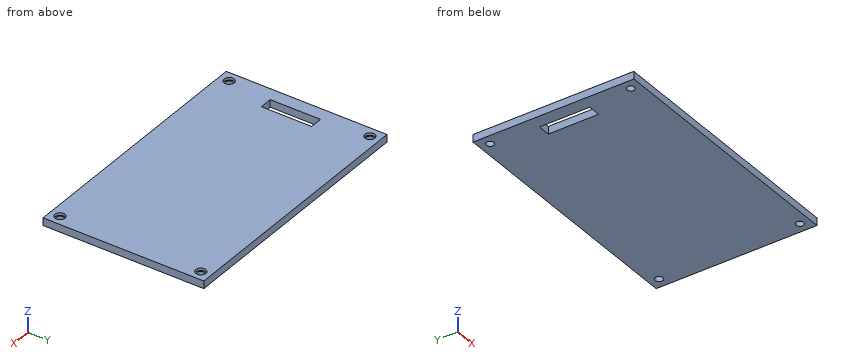
from build123d import *

# Parameters (mm, degrees)
SKETCH_1_W          = 104
SKETCH_1_H          = 64
EXTRUDE_1_DEPTH     = 3
SKETCH_2_R          = 1.5
CUT_EXTRUDE_1_DEPTH = 62.131006862
SKETCH_3_W          = 5
SKETCH_3_H          = 20
CUT_EXTRUDE_2_DEPTH = 62.131006862
SKETCH_4_R          = 2
CUT_EXTRUDE_3_DEPTH = 1


with BuildPart() as part:
    # 草图1 → 凸台-拉伸1 (new body)
    with BuildSketch(Plane.XY):
        Rectangle(SKETCH_1_W, SKETCH_1_H)
    extrude(amount=EXTRUDE_1_DEPTH)

    # 草图2 → 切除-拉伸1 (cut, through all)
    with BuildSketch(Plane.XY.offset(3)):
        with Locations((-48, 28)):
            Circle(SKETCH_2_R)
        with Locations(Location((48, 28, 0), (0, 0, 180))):
            Circle(SKETCH_2_R)
        with Locations((48, -28)):
            Circle(SKETCH_2_R)
        with Locations(Location((-48, -28, 0), (0, 0, 180))):
            Circle(SKETCH_2_R)
    extrude(amount=-CUT_EXTRUDE_1_DEPTH, mode=Mode.SUBTRACT)

    # 草图3 → 切除-拉伸2 (cut, through all)
    with BuildSketch(Plane(origin=(0, 0, 0), x_dir=(-1, 0, 0), z_dir=(0, 0, -1))):
        with Locations((44.26005687, -0.800014708)):
            Rectangle(SKETCH_3_W, SKETCH_3_H)
    extrude(amount=-CUT_EXTRUDE_2_DEPTH, mode=Mode.SUBTRACT)

    # 草图4 → 切除-拉伸3 (cut)
    with BuildSketch(Plane.XY.offset(3)):
        with Locations((48, 28)):
            Circle(SKETCH_4_R)
        with Locations(Location((-48, 28, 0), (0, 0, 180))):
            Circle(SKETCH_4_R)
        with Locations((-48, -28)):
            Circle(SKETCH_4_R)
        with Locations(Location((48, -28, 0), (0, 0, 180))):
            Circle(SKETCH_4_R)
    extrude(amount=-CUT_EXTRUDE_3_DEPTH, mode=Mode.SUBTRACT)


solid = part.part
Verification items for the finished model (mm, model axes). Coordinates: 2 decimals unless noted, no trailing zeros. Order: outer loops, then holes, each group sorted by start corner. A loop starts at its lowest first (then second) coordinate and runs counter-clockwise, first axis right, second up. Notation, with made-up numbers: (-18.75, 69) -> (30.25, 69) arc R18 cw to (30.25, 75) -> close; hole circle Ø8 at (4.5, -24.5). An arc over 180 degrees is marked (long way). Put each result on its own line as item: value. Start each with the question number.
1. Material ranges on L1, parallel to Y at x = 48, z = 1; L2, parallel to Y at x = 48, z = 2.7; L3, parallel to X at y = -2.5, z = 0.85, recorded low to high. Write a range as [from, to].
2. Cross-section at A-A, the plane y = -28. Record the boundary of the cut face in (x, z).
3. Go/stop test with flat-tipped pins: pin 1 Ø1 at (x, y) = (3.5, 13) entering from -Z; pin 2 Ø3.5 at (x, y) = (48, 28) entering from +Z. Record where each tip stops, or that it passes through.
4. Cross-section at C-C, the plane x = -48. Record the boundary of the cut face in (y, z), then the cut area to 3 significant figures.
5. Cross-section at D-D, the plane y = -7. Record the boundary of the cut face in (x, z), then the cut area to 3 significant figures.
6. Cross-section at B-B, the plane z = 1.45. Record the boundary of the cut face in (x, y), then the cut area to 3 significant figures.
Computed:
1. L1: [-32, -29.5], [-26.5, 26.5], [29.5, 32]
1. L2: [-32, -30], [-26, 26], [30, 32]
1. L3: [-52, -46.76], [-41.76, 52]
2. outline: (-52, 0) -> (-49.5, 0) -> (-49.5, 2) -> (-50, 2) -> (-50, 3) -> (-52, 3) -> close; (-46.5, 0) -> (46.5, 0) -> (46.5, 2) -> (46, 2) -> (46, 3) -> (-46, 3) -> (-46, 2) -> (-46.5, 2) -> close; (49.5, 0) -> (52, 0) -> (52, 3) -> (50, 3) -> (50, 2) -> (49.5, 2) -> close
3. pin 1: z = 0
3. pin 2: z = 2
4. outline: (-32, 0) -> (-29.5, 0) -> (-29.5, 2) -> (-30, 2) -> (-30, 3) -> (-32, 3) -> close; (-26.5, 0) -> (26.5, 0) -> (26.5, 2) -> (26, 2) -> (26, 3) -> (-26, 3) -> (-26, 2) -> (-26.5, 2) -> close; (29.5, 0) -> (32, 0) -> (32, 3) -> (30, 3) -> (30, 2) -> (29.5, 2) -> close
4. area: 172 mm2
5. outline: (-52, 0) -> (-46.76, 0) -> (-46.76, 3) -> (-52, 3) -> close; (-41.76, 0) -> (52, 0) -> (52, 3) -> (-41.76, 3) -> close
5. area: 297 mm2
6. outline: (-52, -32) -> (52, -32) -> (52, 32) -> (-52, 32) -> close; hole circle Ø3 at (-48, -28); hole circle Ø3 at (-48, 28); hole (-46.76, -10.8) -> (-41.76, -10.8) -> (-41.76, 9.2) -> (-46.76, 9.2) -> close; hole circle Ø3 at (48, -28); hole circle Ø3 at (48, 28)
6. area: 6,530 mm2
